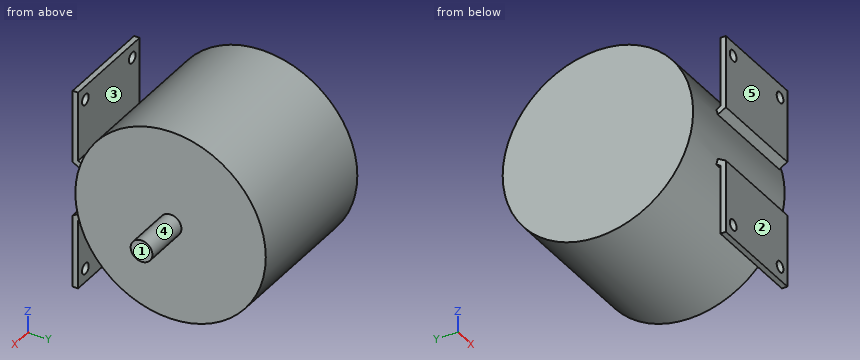
from build123d import *

# Parameters (mm, degrees)
SKETCH1_R           = 52.5
BOSS_EXTRUDE1_DEPTH = 82
SKETCH2_R           = 6
BOSS_EXTRUDE2_DEPTH = 26
BOSS_EXTRUDE3_START = -55
BOSS_EXTRUDE3_DEPTH = 55
CUT_EXTRUDE1_REACH  = 164.336
SKETCH4_R           = 3


with BuildPart() as part:
    # Sketch1 → Boss-Extrude1 (new body)
    with BuildSketch(Plane(origin=(0, 0, 0), x_dir=(0, 0, -1), z_dir=(1, 0, 0))):
        Circle(SKETCH1_R)
    extrude(amount=BOSS_EXTRUDE1_DEPTH)

    # Sketch2 → Boss-Extrude2 (add)
    with BuildSketch(Plane(origin=(82, 0, 0), x_dir=(0, 0, -1), z_dir=(1, 0, 0))):
        with Locations(Location((0, 0, 0), (0, 0, 180))):
            Circle(SKETCH2_R)
    extrude(amount=BOSS_EXTRUDE2_DEPTH)

    # Sketch3 → Boss-Extrude3 (add)
    with BuildSketch(Plane(origin=(79.5, 0, 0), x_dir=(0, 0, -1), z_dir=(1, 0, 0)).offset(BOSS_EXTRUDE3_START)):
        with BuildLine():
            Line((-55, -52.5), (-16.732050808, -52.5))
            Line((-16.732050808, -52.5), (-15.398880082, -50.190880568))
            ThreePointArc((-15.398880082, -50.190880568), (-13.910046874, -50.623715746), (-12.409081478, -51.012397482))
            Line((-12.409081478, -51.012397482), (-15, -55.5))
            Line((-15, -55.5), (-55, -55.5))
            Line((-55, -55.5), (-55, -52.5))
        make_face()
        with BuildLine():
            Line((16.732050808, -52.5), (15.398880082, -50.190880568))
            ThreePointArc((15.398880082, -50.190880568), (13.910046874, -50.623715746), (12.409081478, -51.012397482))
            Line((12.409081478, -51.012397482), (15, -55.5))
            Line((15, -55.5), (55, -55.5))
            Line((55, -55.5), (55, -52.5))
            Line((55, -52.5), (16.732050808, -52.5))
        make_face()
    extrude(amount=BOSS_EXTRUDE3_DEPTH)

    # Sketch4 → Cut-Extrude1 (cut, up to next)
    with BuildSketch(Plane.XZ.offset(55.5), mode=Mode.PRIVATE) as cut_extrude1_sk1:
        with Locations(Location((73, 47.5, 0), (0, 0, 270))):
            Circle(SKETCH4_R)
    cut_extrude1_tool1 = extrude(cut_extrude1_sk1.sketch, amount=-CUT_EXTRUDE1_REACH, mode=Mode.PRIVATE) & part.part
    # Sketch4 → Cut-Extrude1 (cut, up to next)
    with BuildSketch(Plane.XZ.offset(55.5), mode=Mode.PRIVATE) as cut_extrude1_sk2:
        with Locations(Location((73, -47.5, 0), (0, 0, 90))):
            Circle(SKETCH4_R)
    cut_extrude1_tool2 = extrude(cut_extrude1_sk2.sketch, amount=-CUT_EXTRUDE1_REACH, mode=Mode.PRIVATE) & part.part
    # Sketch4 → Cut-Extrude1 (cut, up to next)
    with BuildSketch(Plane.XZ.offset(55.5), mode=Mode.PRIVATE) as cut_extrude1_sk3:
        with Locations(Location((31, -47.5, 0), (0, 0, 90))):
            Circle(SKETCH4_R)
    cut_extrude1_tool3 = extrude(cut_extrude1_sk3.sketch, amount=-CUT_EXTRUDE1_REACH, mode=Mode.PRIVATE) & part.part
    # Sketch4 → Cut-Extrude1 (cut, up to next)
    with BuildSketch(Plane.XZ.offset(55.5), mode=Mode.PRIVATE) as cut_extrude1_sk4:
        with Locations(Location((31, 47.5, 0), (0, 0, 270))):
            Circle(SKETCH4_R)
    cut_extrude1_tool4 = extrude(cut_extrude1_sk4.sketch, amount=-CUT_EXTRUDE1_REACH, mode=Mode.PRIVATE) & part.part
    add(cut_extrude1_tool1.solids().sort_by_distance((73, -55.5, 47.5))[0], mode=Mode.SUBTRACT)
    add(cut_extrude1_tool2.solids().sort_by_distance((73, -55.5, -47.5))[0], mode=Mode.SUBTRACT)
    add(cut_extrude1_tool3.solids().sort_by_distance((31, -55.5, -47.5))[0], mode=Mode.SUBTRACT)
    add(cut_extrude1_tool4.solids().sort_by_distance((31, -55.5, 47.5))[0], mode=Mode.SUBTRACT)


solid = part.part
Can you work these out from the model? Positions are in its coordinate system, mm. Face numbers are marked on the shaded views. A direction names the side the tool comes from. Round coordinates to 2 decimals unless told otherwise and drop trailing zeros. Write each loop counter-clockwise with the first axis right and the second up, starting at its lowest first coordinate (ties: lowest second). Pieces come first, ordered by that corner, then holes. Notation, with made-up numbers: (56, 58.25) - (103, 58.25) arc R22 ccw to (103, 82.25) - close; hole circle Ø10 at (-27.75, 55). An arc over 180 degrees is marked (long way). Write each question's results on one line, items separated by ' | '. Start each with the question number.
1) Suppose I cut it at B-B (z = 47.5). List the corners of the cut face in (x, y) for me, and give its area (3 significant figures).
2) Suppose I cut it at C-C (y = 0). List the corners of the cut face in (x, z) for me, and give its area (3 significant figures).
3) We'd pull the mould along Y, two halves only. Please class the marked faces 1, 2 and 3: released by +Y, released by -Y, zero draft, split by the parting line, or undercut.
4) Suppose I cut it at D-D (z = -37). List the corners of the cut face in (x, y) for me, and give its area (3 significant figures).
5) Suppose I cut it at A-A (x = 54). List the corners of the cut face in (y, z) for me.
6) Please list where these lines run through material, in increasing order: line 1 (X direction, y = -54, z = -47); line 2 (X direction, y = -12.5, z = 38.5); line 3 (Y direction, x = 46, z = -38.5).
7) For pin 1 Ø7 at (x, z) = (31, 47.5) entering from +Y; pin 2 Ø3.5 at (x, z) = (73, -47.5) entering from -Y; pin 3 Ø12 at (x, y) = (33.5, 25) entering from -Z, each with a flat end and sliding along its axis, tell me the tip position at first contact or that it passes through.
8) Which directions (+Z, -Z, +X, -X, +Y, -Y) give clear straight access to the entire face, cutting with the end or side of a thin tool? Please do the marked faces 4 and 5.
Here are the results:
1) outline: (0, -22.36) - (82, -22.36) - (82, 22.36) - (0, 22.36) - close; (24.5, -55.5) - (28, -55.5) - (28, -52.5) - (24.5, -52.5) - close; (34, -55.5) - (70, -55.5) - (70, -52.5) - (34, -52.5) - close; (76, -55.5) - (79.5, -55.5) - (79.5, -52.5) - (76, -52.5) - close | area: 3,800 mm2
2) outline: (0, -52.5) - (82, -52.5) - (82, -6) - (108, -6) - (108, 6) - (82, 6) - (82, 52.5) - (0, 52.5) - close | area: 8,920 mm2
3) face 1: zero draft | face 2: released by -Y | face 3: undercut
4) outline: (0, -37.25) - (82, -37.25) - (82, 37.25) - (0, 37.25) - close; (24.5, -55.5) - (79.5, -55.5) - (79.5, -52.5) - (24.5, -52.5) - close | area: 6,270 mm2
5) outline: (-55.5, -55) - (-52.5, -55) - (-52.5, -16.73) - (-50.19, -15.4) arc R52.5 ccw (long way) to (-50.19, 15.4) - (-52.5, 16.73) - (-52.5, 55) - (-55.5, 55) - (-55.5, 15) - (-51.01, 12.41) arc R52.5 ccw to (-51.01, -12.41) - (-55.5, -15) - close
6) line 1: x = 24.5 to 28.04, 33.96 to 70.04, 75.96 to 79.5 | line 2: x = 0 to 82 | line 3: y = -55.5 to -52.5, -35.69 to 35.69
7) pin 1: stops at y = 28.64 | pin 2: stops at y = -25.75 | pin 3: stops at z = -48.94
8) face 4: +X | face 5: +Z, -Z, +X, -X, -Y
